Could you check a few things on this model? Use its own coordinates, in mm. A direction names the side the tool comes from. Coordinates: 2 decimals unless noted, no trailing zeros. Order: outer loops, then holes, each group sorted by start corner. A loop starts at its lowest first (then second) coordinate and runs counter-clockwise, first axis right, second up. Notation, with made-up numbers: (-28.5, 47) - (0.5, 47) arc R24 cw to (0.5, 61) - close; hole circle Ø10 at (20.25, 30.25). An arc over 180 degrees is marked (long way). One line per item, written item: value.
from build123d import *

# Parameters (mm, degrees)
SKETCH2_W           = 398.100558659
SKETCH2_H           = 70
BOSS_EXTRUDE1_DEPTH = 20
CUT_EXTRUDE1_DEPTH  = 10


with BuildPart() as part:
    # Sketch2 → Boss-Extrude1 (new body)
    with BuildSketch(Plane(origin=(0, 0, 0), x_dir=(0, 0, -1), z_dir=(1, 0, 0))):
        with Locations((199.05027933, 35)):
            Rectangle(SKETCH2_W, SKETCH2_H)
    extrude(amount=BOSS_EXTRUDE1_DEPTH)

    # Sketch3 → Cut-Extrude1 (cut)
    with BuildSketch(Plane(origin=(20, 0, 0), x_dir=(0, 0, -1), z_dir=(1, 0, 0))):
        with BuildLine():
            Line((35, 52.5), (363.100558659, 52.5))
            ThreePointArc((363.100558659, 52.5), (380.600558659, 35), (363.100558659, 17.5))
            Line((363.100558659, 17.5), (35, 17.5))
            ThreePointArc((35, 17.5), (17.5, 35), (35, 52.5))
        make_face()
    extrude(amount=-CUT_EXTRUDE1_DEPTH, mode=Mode.SUBTRACT)


solid = part.part
Item 1: I want a section at B-B on y = 35. Please give me the cut outline in (x, z).
Conclusion:
outline: (0, -398.1) - (20, -398.1) - (20, -380.6) - (10, -380.6) - (10, -17.5) - (20, -17.5) - (20, 0) - (0, 0) - close
Item 2: If I drill on probe 1 along Y at (x, z) = (10.5, -299.5); probe 2 along Z at (x, y) = (13.5, 48); probe 3 along X at (y, z) = (45.5, -207), over which ranges is the centre line in solid material (lowest first)?
Conclusion:
probe 1: 0 to 17.5, 52.5 to 70
probe 2: -398.1 to -374.82, -23.28 to 0
probe 3: 0 to 10
Item 3: Thinking about a two-plate mould opening in Z: for faces 1 (the face through (10, 35, -398.101)), 2 (the face through (15.07, 35.385, -380.596)), 3 (the face through (0, 35, -196)), which applies, pulls with the +Z half, pulls with the -Z half, needs draft (parallel to the pull), parting line crosses it, or undercut?
Conclusion:
face 1: pulls with the -Z half
face 2: undercut
face 3: needs draft
Item 4: I want a section at A-A on z = -210.5. Please give me the cut outline in (x, y), then the cut area to 3 significant figures.
Conclusion:
outline: (0, 0) - (20, 0) - (20, 17.5) - (10, 17.5) - (10, 52.5) - (20, 52.5) - (20, 70) - (0, 70) - close
area: 1,050 mm²
Item 5: I'm going to push flat-ended pins straight in: pin 1 Ø6 at (x, z) = (10, -153) entering from -Y; pin 2 Ø10.5 at (y, z) = (28.5, -153) entering from +X. Where does each tip first touch, or does it pass through?
Conclusion:
pin 1: y = 0
pin 2: x = 10
Item 6: For faces 4 (the face through (10, 35, -202)), 5 (the face through (20, 59, -196)), which set-ups out of +Z, -Z, +X, -X, +Y, -Y let a thin tool reach every point of the face, with its end or its side?
Conclusion:
face 4: +X
face 5: +Z, -Z, +X, +Y, -Y
